Here's how the part is built. I have some questions about the finished solid (model axes, mm). A direction names the side the tool comes from. Coordinates: 2 decimals unless noted, no trailing zeros. Write each loop counter-clockwise with the first axis right and the second up, starting at its lowest first coordinate (ties: lowest second). Pieces come first, ordered by that corner, then holes. Notation, with made-up numbers: (54.5, 43.25) -> (109.5, 43.25) arc R19 ccw to (109.5, 73.25) -> close; hole circle Ø5 at (35.25, 15). An arc over 180 degrees is marked (long way). Use a Markdown table: item, result. Add a question column.
Item 1: Imagine slicing it at A-A, the plane y = -4. Write out the boundary of the cut face in (x, z) (3 decimals), and give its area (3 significant figures).
Item 2: If we mould it in two halves opening along Z, with no side actions, what happens to faces 4 (the cylindrical face through (4.69, 7, 3.92)), 5 (the cylindrical face through (2.272, 7.273, 0.336)), 6 (the cylindrical face through (-0.251, 7.311, 6.194)), 7 (the flat face through (1.12, 3.84, 3.9))? For each: pulls with the +Z half, pulls with the -Z half, needs draft (parallel to the pull), parting line crosses it, or undercut.
Item 3: On a 3-axis mill with a long thin cutter (end or side, diameter ignored), from which of +Z, -Z, +X, -X, +Y, -Y can I reach the whole of each face in a straight line? I mean faces 1 (the flat face through (-2, -7, 2.925)), 2 (the flat face through (1.355, 8.005, 5.579)), 3 (the cylindrical face through (2.26, -6.97, 1.59)). Say none if no direction works.
Item 4: If I drill on line 1 along Y through (x, z) = (0, 0.3); line 2 along Z through (x, y) = (0, -8) (3 decimals); line 3 along X through (y, z) = (-1.5, 3.5), over which ranges is the centre line in solid material (lowest first)? Write a range as from..to.
Item 5: Will these pins go through, and if not, where does the flat tip stop? pin 1 Ø4 at (x, y) = (1, 9) entering from -Z (3 decimals); pin 2 Ø1 at (x, y) = (1.5, -6) entering from -Z; pin 3 Ø1.8 at (x, y) = (1, 6.5) entering from +Z.
```python
from build123d import *

# Parameters (mm, degrees)
CROQUIS1_R                   = 3.6
CROQUIS1_R_2                 = 3.1
SALIENTE_EXTRUIR1_DEPTH      = 7.87
SALIENTE_EXTRUIR2_START      = 0.85
CROQUIS1_3_R                 = 3.1
CROQUIS1_3_R_2               = 2.475
SALIENTE_EXTRUIR2_DEPTH      = 6.17
SALIENTE_EXTRUIR3_REACH      = 13.518
SALIENTE_EXTRUIR3_END_RADIUS = 3.6
SALIENTE_EXTRUIR4_START      = -8
SALIENTE_EXTRUIR4_DEPTH      = 8
SALIENTE_EXTRUIR5_REACH      = 20.306
SALIENTE_EXTRUIR5_END_RADIUS = 3.6
SALIENTE_EXTRUIR6_START      = -8
SALIENTE_EXTRUIR6_DEPTH      = 8


with BuildPart() as part:
    # Croquis1 → Saliente-Extruir1 (new body)
    with BuildSketch(Plane.XY):
        Circle(CROQUIS1_R)
        Circle(CROQUIS1_R_2, mode=Mode.SUBTRACT)
    extrude(amount=SALIENTE_EXTRUIR1_DEPTH)

    # Croquis1<3> → Saliente-Extruir2 (add)
    with BuildSketch(Plane.XY.offset(SALIENTE_EXTRUIR2_START)):
        Circle(CROQUIS1_3_R)
        Circle(CROQUIS1_3_R_2, mode=Mode.SUBTRACT)
    extrude(amount=SALIENTE_EXTRUIR2_DEPTH)

    # Saliente-Extruir3: up to this cylinder (the profile starts outside it)
    saliente_extruir3_end = Plane(origin=(0, 0, 6.19961), z_dir=(0, 0, -1)) * Cylinder(SALIENTE_EXTRUIR3_END_RADIUS, 35.236000000000004, mode=Mode.PRIVATE)
    # Croquis2 → Saliente-Extruir3 (add, up to the surface)
    with BuildSketch(Plane(origin=(0, -4, 0), x_dir=(1, 0, 0), z_dir=(0, 1, 0)), mode=Mode.PRIVATE) as saliente_extruir3_sk1:
        with BuildLine():
            ThreePointArc((-1.7124779696357202, -7.101610049171246), (0.05399392602494436, -7.534595068330939), (1.806684459564255, -7.048822612733265))
            ThreePointArc((1.806684459564255, -7.048822612733265), (2.337681630948243, -6.203587592595142), (3.1666100491712275, -5.647477969635754))
            ThreePointArc((3.1666100491712275, -5.647477969635754), (3.599595068330938, -3.881006073975069), (3.1138226127332604, -2.1283155404357355))
            ThreePointArc((3.1138226127332604, -2.1283155404357355), (2.268587592595135, -1.597318369051751), (1.7124779696357444, -0.7683899508287686))
            ThreePointArc((1.7124779696357444, -0.7683899508287686), (-0.0539939260249431, -0.3354049316690628), (-1.806684459564274, -0.8211773872667488))
            ThreePointArc((-1.806684459564274, -0.8211773872667488), (-2.337681630948256, -1.6664124074048765), (-3.166610049171237, -2.22252203036427))
            ThreePointArc((-3.166610049171237, -2.22252203036427), (-3.599595068330935, -3.9889939260249565), (-3.1138226127332462, -5.741684459564288))
            ThreePointArc((-3.1138226127332462, -5.741684459564288), (-2.268587592595116, -6.272681630948267), (-1.7124779696357202, -7.101610049171246))
        make_face()
        with BuildLine():
            Line((-1.01, -6.194540882568846), (-1.01, -4.944999999999999))
            Line((-1.01, -4.944999999999999), (-2.2595408825688463, -4.944999999999999))
            ThreePointArc((-2.2595408825688463, -4.944999999999999), (-2.475, -3.9349999999999996), (-2.2595408825688463, -2.9250000000000007))
            Line((-2.2595408825688463, -2.9250000000000007), (-1.01, -2.9250000000000007))
            Line((-1.01, -2.9250000000000007), (-1.01, -1.675459117431154))
            ThreePointArc((-1.01, -1.675459117431154), (1.5e-16, -1.4600000000000004), (1.01, -1.675459117431154))
            Line((1.01, -1.675459117431154), (1.01, -2.9250000000000007))
            Line((1.01, -2.9250000000000007), (2.2595408825688463, -2.9250000000000007))
            ThreePointArc((2.2595408825688463, -2.9250000000000007), (2.475, -3.935), (2.2595408825688463, -4.944999999999999))
            Line((2.2595408825688463, -4.944999999999999), (1.01, -4.944999999999999))
            Line((1.01, -4.944999999999999), (1.01, -6.194540882568846))
            ThreePointArc((1.01, -6.194540882568846), (1.5e-16, -6.41), (-1.01, -6.194540882568846))
        make_face(mode=Mode.SUBTRACT)
    saliente_extruir3_tool1 = extrude(saliente_extruir3_sk1.sketch, amount=SALIENTE_EXTRUIR3_REACH, mode=Mode.PRIVATE) - saliente_extruir3_end
    add(saliente_extruir3_tool1.solids().sort_by_distance((-2.197676, -4, 6.19961))[0])

    # Croquis2<3> → Saliente-Extruir4 (add)
    with BuildSketch(Plane(origin=(0, -4, 0), x_dir=(1, 0, 0), z_dir=(0, 1, 0)).offset(SALIENTE_EXTRUIR4_START)):
        with BuildLine():
            ThreePointArc((-3.166610049171237, -2.22252203036427), (-2.337681630948256, -1.6664124074048765), (-1.806684459564274, -0.8211773872667488))
            ThreePointArc((-1.806684459564274, -0.8211773872667488), (-0.0539939260249431, -0.3354049316690628), (1.7124779696357444, -0.7683899508287686))
            ThreePointArc((1.7124779696357444, -0.7683899508287686), (2.268587592595135, -1.597318369051751), (3.1138226127332604, -2.1283155404357355))
            ThreePointArc((3.1138226127332604, -2.1283155404357355), (3.599595068330938, -3.881006073975069), (3.1666100491712275, -5.647477969635754))
            ThreePointArc((3.1666100491712275, -5.647477969635754), (2.337681630948243, -6.203587592595142), (1.806684459564255, -7.048822612733265))
            ThreePointArc((1.806684459564255, -7.048822612733265), (0.05399392602494436, -7.534595068330939), (-1.7124779696357202, -7.101610049171246))
            ThreePointArc((-1.7124779696357202, -7.101610049171246), (-2.268587592595116, -6.272681630948267), (-3.1138226127332462, -5.741684459564288))
            ThreePointArc((-3.1138226127332462, -5.741684459564288), (-3.599595068330935, -3.9889939260249565), (-3.166610049171237, -2.22252203036427))
        make_face()
        with BuildLine():
            ThreePointArc((-2.2595408825688463, -2.9250000000000007), (-2.475, -3.9349999999999996), (-2.2595408825688463, -4.944999999999999))
            Line((-2.2595408825688463, -4.944999999999999), (-1.01, -4.944999999999999))
            Line((-1.01, -4.944999999999999), (-1.01, -6.194540882568846))
            ThreePointArc((-1.01, -6.194540882568846), (1.5e-16, -6.41), (1.01, -6.194540882568846))
            Line((1.01, -6.194540882568846), (1.01, -4.944999999999999))
            Line((1.01, -4.944999999999999), (2.2595408825688463, -4.944999999999999))
            ThreePointArc((2.2595408825688463, -4.944999999999999), (2.475, -3.935), (2.2595408825688463, -2.9250000000000007))
            Line((2.2595408825688463, -2.9250000000000007), (1.01, -2.9250000000000007))
            Line((1.01, -2.9250000000000007), (1.01, -1.675459117431154))
            ThreePointArc((1.01, -1.675459117431154), (1.5e-16, -1.4600000000000004), (-1.01, -1.675459117431154))
            Line((-1.01, -1.675459117431154), (-1.01, -2.9250000000000007))
            Line((-1.01, -2.9250000000000007), (-2.2595408825688463, -2.9250000000000007))
        make_face(mode=Mode.SUBTRACT)
    extrude(amount=SALIENTE_EXTRUIR4_DEPTH)

    # Saliente-Extruir5: up to this cylinder (the profile starts outside it)
    saliente_extruir5_end = Plane(origin=(0, 0, 3.935), z_dir=(0, 0, -1)) * Cylinder(SALIENTE_EXTRUIR5_END_RADIUS, 48.812000000000005, mode=Mode.PRIVATE)
    # Croquis7 → Saliente-Extruir5 (add, up to the surface)
    with BuildSketch(Plane(origin=(1.152785072536334, 3.830285443219265, 0), x_dir=(0, 0, 1), z_dir=(-0.2881962681340835, -0.9575713608048162, 0)), mode=Mode.PRIVATE) as saliente_extruir5_sk1:
        with BuildLine():
            ThreePointArc((2.222522030364279, -3.1666100491712452), (3.9889939260249445, -3.5995950683309377), (5.741684459564254, -3.113822612733264))
            ThreePointArc((5.741684459564254, -3.113822612733264), (6.272681630948287, -2.2685875925951686), (7.101610049171227, -1.7124779696357533))
            ThreePointArc((7.101610049171227, -1.7124779696357533), (7.534595068330938, 0.0539939260249318), (7.048822612733259, 1.8066844595642648))
            ThreePointArc((7.048822612733259, 1.8066844595642648), (6.203587592595132, 2.337681630948248), (5.647477969635745, 3.1666100491712332))
            ThreePointArc((5.647477969635745, 3.1666100491712332), (3.881006073975058, 3.599595068330939), (2.1283155404357252, 3.113822612733254))
            ThreePointArc((2.1283155404357252, 3.113822612733254), (1.5973183690517558, 2.268587592595114), (0.7683899508287607, 1.7124779696357326))
            ThreePointArc((0.7683899508287607, 1.7124779696357326), (0.33540493166906193, -0.05399392602495561), (0.8211773872667536, -1.8066844595642866))
            ThreePointArc((0.8211773872667536, -1.8066844595642866), (1.6664124074048823, -2.337681630948267), (2.222522030364279, -3.1666100491712452))
        make_face()
    saliente_extruir5_tool1 = extrude(saliente_extruir5_sk1.sketch, amount=SALIENTE_EXTRUIR5_REACH, mode=Mode.PRIVATE) - saliente_extruir5_end
    add(saliente_extruir5_tool1.solids().sort_by_distance((1.152785, 3.830285, 3.935))[0])

    # Croquis7<3> → Saliente-Extruir6 (add)
    with BuildSketch(Plane(origin=(1.152785072536334, 3.830285443219265, 0), x_dir=(0, 0, 1), z_dir=(-0.2881962681340835, -0.9575713608048162, 0)).offset(SALIENTE_EXTRUIR6_START)):
        with BuildLine():
            ThreePointArc((0.7683899508287607, 1.7124779696357326), (1.5973183690517558, 2.268587592595114), (2.1283155404357252, 3.113822612733254))
            ThreePointArc((2.1283155404357252, 3.113822612733254), (3.881006073975058, 3.599595068330939), (5.647477969635745, 3.1666100491712332))
            ThreePointArc((5.647477969635745, 3.1666100491712332), (6.203587592595132, 2.337681630948248), (7.048822612733259, 1.8066844595642648))
            ThreePointArc((7.048822612733259, 1.8066844595642648), (7.534595068330938, 0.0539939260249318), (7.101610049171227, -1.7124779696357533))
            ThreePointArc((7.101610049171227, -1.7124779696357533), (6.272681630948287, -2.2685875925951686), (5.741684459564254, -3.113822612733264))
            ThreePointArc((5.741684459564254, -3.113822612733264), (3.9889939260249445, -3.5995950683309377), (2.222522030364279, -3.1666100491712452))
            ThreePointArc((2.222522030364279, -3.1666100491712452), (1.6664124074048823, -2.337681630948267), (0.8211773872667536, -1.8066844595642866))
            ThreePointArc((0.8211773872667536, -1.8066844595642866), (0.33540493166906193, -0.05399392602495561), (0.7683899508287607, 1.7124779696357326))
        make_face()
        with BuildLine():
            ThreePointArc((1.675459117431154, 1.010000000000001), (1.4600000000000004, 1.17e-15), (1.675459117431154, -1.0099999999999991))
            Line((1.675459117431154, -1.0099999999999991), (2.925, -1.0099999999999991))
            Line((2.925, -1.0099999999999991), (2.925, -2.2595408825688454))
            ThreePointArc((2.925, -2.2595408825688454), (3.934999999999999, -2.474999999999999), (4.944999999999999, -2.259540882568846))
            Line((4.944999999999999, -2.259540882568846), (4.944999999999999, -1.009999999999999))
            Line((4.944999999999999, -1.009999999999999), (6.194540882568846, -1.0099999999999987))
            ThreePointArc((6.194540882568846, -1.0099999999999987), (6.41, 1e-15), (6.194540882568846, 1.010000000000001))
            Line((6.194540882568846, 1.010000000000001), (4.944999999999999, 1.010000000000001))
            Line((4.944999999999999, 1.010000000000001), (4.944999999999999, 2.259540882568847))
            ThreePointArc((4.944999999999999, 2.259540882568847), (3.9349999999999996, 2.475000000000001), (2.925, 2.2595408825688468))
            Line((2.925, 2.2595408825688468), (2.925, 1.010000000000001))
            Line((2.925, 1.010000000000001), (1.675459117431154, 1.010000000000001))
        make_face(mode=Mode.SUBTRACT)
    extrude(amount=SALIENTE_EXTRUIR6_DEPTH)


solid = part.part
```
Ans:
| question | item | result |
|---|---|---|
| 1 | outline | (-3.167, 2.223) arc R2.4 cw to (-1.807, 0.821) arc R3.6 ccw to (1.712, 0.768) arc R2.4 cw to (3.114, 2.128) arc R3.6 ccw to (3.167, 5.647) arc R2.4 cw to (1.807, 7.049) arc R3.6 ccw to (-1.712, 7.102) arc R2.4 cw to (-3.114, 5.742) arc R3.6 ccw to start; hole (-2.26, 2.925) -> (-1.01, 2.925) -> (-1.01, 1.675) arc R2.475 ccw to (1.01, 1.675) -> (1.01, 2.925) -> (2.26, 2.925) arc R2.475 ccw to (2.26, 4.945) -> (1.01, 4.945) -> (1.01, 6.195) arc R2.475 ccw to (-1.01, 6.195) -> (-1.01, 4.945) -> (-2.26, 4.945) arc R2.475 ccw to start |
| 1 | area | 23.6 mm^2 |
| 2 | face 4 | undercut |
| 2 | face 5 | pulls with the -Z half |
| 2 | face 6 | pulls with the +Z half |
| 2 | face 7 | undercut |
| 3 | face 1 | -Y |
| 3 | face 2 | none |
| 3 | face 3 | -Z, +X, -Y |
| 4 | line 1 | y = -3.6..-3.1, 3.1..3.6 |
| 4 | line 2 | z = 0.335..1.46, 6.41..7.535 |
| 4 | line 3 | x = -3.57..-1.97, 1.97..3.57 |
| 5 | pin 1 | stops at z = 0.335 |
| 5 | pin 2 | stops at z = 0.48 |
| 5 | pin 3 | stops at z = 7.53 |
